```python
from build123d import *

# Parameters (mm, degrees)
BOSS_EXTRUDE1_DEPTH = 518.16
SKETCH2_R           = 4.7625
CUT_EXTRUDE1_DEPTH  = 520.304779053


with BuildPart() as part:
    # Sketch1 → Boss-Extrude1 (new body)
    with BuildSketch(Plane.XY):
        with BuildLine():
            Line((-0.8382, 23.2918), (22.0218, 23.2918))
            ThreePointArc((22.0218, 23.2918), (22.919825612, 22.919825612), (23.2918, 22.0218))
            Line((23.2918, 22.0218), (23.2918, -0.8382))
            ThreePointArc((23.2918, -0.8382), (22.919825612, -1.736225612), (22.0218, -2.1082))
            Line((22.0218, -2.1082), (-0.8382, -2.1082))
            ThreePointArc((-0.8382, -2.1082), (-1.736225612, -1.736225612), (-2.1082, -0.8382))
            Line((-2.1082, -0.8382), (-2.1082, 22.0218))
            ThreePointArc((-2.1082, 22.0218), (-1.736225612, 22.919825612), (-0.8382, 23.2918))
        make_face()
        with BuildLine():
            Line((1.27, 0), (19.9136, 0))
            ThreePointArc((19.9136, 0), (20.811625612, 0.371974388), (21.1836, 1.27))
            Line((21.1836, 1.27), (21.1836, 19.9136))
            ThreePointArc((21.1836, 19.9136), (20.811625612, 20.811625612), (19.9136, 21.1836))
            Line((19.9136, 21.1836), (1.27, 21.1836))
            ThreePointArc((1.27, 21.1836), (0.371974388, 20.811625612), (0, 19.9136))
            Line((0, 19.9136), (0, 1.27))
            ThreePointArc((0, 1.27), (0.371974388, 0.371974388), (1.27, 0))
        make_face(mode=Mode.SUBTRACT)
    extrude(amount=BOSS_EXTRUDE1_DEPTH)

    # Sketch2 → Cut-Extrude1 (cut, through all)
    with BuildSketch(Plane.ZY.offset(2.1082)):
        with Locations(Location((259.08, 10.5918, 0), (0, 0, 270))):
            Circle(SKETCH2_R)
    extrude(amount=-CUT_EXTRUDE1_DEPTH, mode=Mode.SUBTRACT)


solid = part.part
```
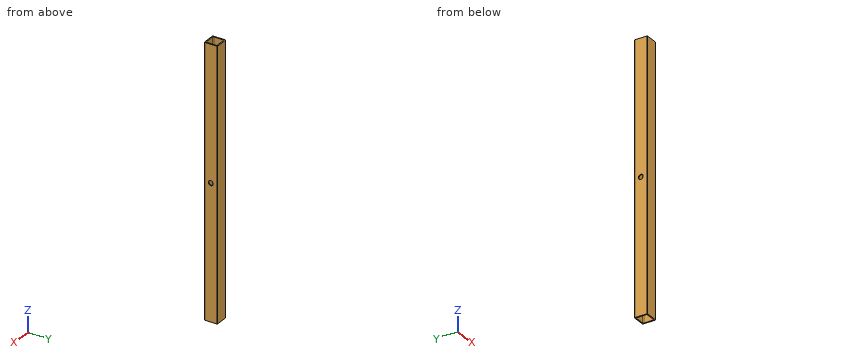
Source: CAD feature listing. Evaluate the final solid. Frame: model axes, mm. Coordinates: 2 decimals unless noted, no trailing zeros. Write each loop counter-clockwise with the first axis right and the second up, starting at its lowest first coordinate (ties: lowest second). Pieces come first, ordered by that corner, then holes. Notation, with made-up numbers: (75.5, 21) - (127.5, 21) arc R21 cw to (127.5, 29) - close; hole circle Ø5 at (18.5, 37). An arc over 180 degrees is marked (long way). Answer as a JSON object with one key per item and string values.
Q1. First-contact query: pin 1 Ø10 at (x, y) = (5.5, 11.5) entering from +Z. Flat tip, straight axial feed; report the tip coordinate or a pass-through.
Ans:
{"pin 1": "passes through"}
Q2. Material intervals for line 1 (Y direction, x = 10.75, z = 220); line 2 (Y direction, x = -0.8, z = 259.08), sorted ascending. Write a range as [from, to].
Ans:
{"line 1": "y = [-2.11, 0], [21.18, 23.29]", "line 2": "y = [-2.11, 5.83], [15.35, 23.29]"}
Q3. Section query B-B, the plane z = 172. Output: boundary loops of the cut face in (x, y), plus the area to 3 significant figures.
Ans:
{"outline": "(-2.11, -0.84) arc R1.27 ccw to (-0.84, -2.11) - (22.02, -2.11) arc R1.27 ccw to (23.29, -0.84) - (23.29, 22.02) arc R1.27 ccw to (22.02, 23.29) - (-0.84, 23.29) arc R1.27 ccw to (-2.11, 22.02) - close; hole (0, 1.27) arc R1.27 ccw to (1.27, 0) - (19.91, 0) arc R1.27 ccw to (21.18, 1.27) - (21.18, 19.91) arc R1.27 ccw to (19.91, 21.18) - (1.27, 21.18) arc R1.27 ccw to (0, 19.91) - close", "area": "196 mm2"}
Q4. Section query A-A, the plane x = 7.5. Output: boundary loops of the cut face in (y, z), plus the area to 3 significant figures.
Ans:
{"outline": "(-2.11, 0) - (0, 0) - (0, 518.16) - (-2.11, 518.16) - close; (21.18, 0) - (23.29, 0) - (23.29, 518.16) - (21.18, 518.16) - close", "area": "2,180 mm2"}
Q5. Section query C-C, the plane z = 259.08. Output: boundary loops of the cut face in (x, y).
Ans:
{"outline": "(-2.11, -0.84) arc R1.27 ccw to (-0.84, -2.11) - (22.02, -2.11) arc R1.27 ccw to (23.29, -0.84) - (23.29, 5.83) - (21.18, 5.83) - (21.18, 1.27) arc R1.27 cw to (19.91, 0) - (1.27, 0) arc R1.27 cw to (0, 1.27) - (0, 5.83) - (-2.11, 5.83) - close; (-2.11, 15.35) - (0, 15.35) - (0, 19.91) arc R1.27 cw to (1.27, 21.18) - (19.91, 21.18) arc R1.27 cw to (21.18, 19.91) - (21.18, 15.35) - (23.29, 15.35) - (23.29, 22.02) arc R1.27 ccw to (22.02, 23.29) - (-0.84, 23.29) arc R1.27 ccw to (-2.11, 22.02) - close"}
